```python
from build123d import *

# Parameters (mm, degrees)
BOSS_EXTRUDE1_DEPTH       = 8
SKETCH2_W                 = 5
SKETCH2_H                 = 5
LPATTERN1_COUNT           = 2
LPATTERN1_PITCH           = 20
LPATTERN1_COL_COUNT       = 2
LPATTERN1_COL_PITCH       = 20
LPATTERN2_COUNT           = 2
LPATTERN2_PITCH           = 25
LPATTERN2_COPY_1_SKETCH_W = 5
LPATTERN2_COPY_1_SKETCH_H = 5
LPATTERN2_COPY_2_SKETCH_W = 5
LPATTERN2_COPY_2_SKETCH_H = 5
SKETCH3_W                 = 30
SKETCH3_H                 = 40
CUT_EXTRUDE1_DEPTH        = 3
FILLET1_R                 = 5
CHAMFER1_SIZE             = 1
SKETCH4_R                 = 1.5
SKETCH4_R_2               = 2.5
CUT_EXTRUDE2_DEPTH        = 131.748804966
SKETCH5_W                 = 12
SKETCH5_H                 = 12
CUT_EXTRUDE3_DEPTH        = 3
FILLET2_R                 = 5


with BuildPart() as part:
    # Sketch1 → Boss-Extrude1 (new body)
    with BuildSketch(Plane(origin=(0, 0, 0), x_dir=(1, 0, 0), z_dir=(0, 1, 0))):
        Polygon((-37.5, 0), (37.5, 0), (37.5, 100), (0, 125), (-37.5, 100), align=None)
    extrude(amount=BOSS_EXTRUDE1_DEPTH)

    # Sketch2 → Revolve1 (revolve)
    with BuildSketch(Plane(origin=(0, 0, 0), x_dir=(0, 0, -1), z_dir=(1, 0, 0)), mode=Mode.PRIVATE) as revolve1_sk:
        with Locations((17.5, 10.5)):
            Rectangle(SKETCH2_W, SKETCH2_H)
    revolve1 = revolve(revolve1_sk.sketch.rotate(Axis((0, 8, -20), (0, 1, 0)), 180), axis=Axis((0, 8, -20), (0, 1, 0)))

    # LPattern1: Revolve1 ×2
    with Locations(*[(-i * LPATTERN1_PITCH, 0, 0) for i in range(1, LPATTERN1_COUNT)]):
        add(revolve1)

    # LPattern1 col: Revolve1 ×2
    with Locations(*[(i * LPATTERN1_COL_PITCH, 0, 0) for i in range(1, LPATTERN1_COL_COUNT)]):
        add(revolve1)

    # LPattern2: Revolve1 ×2
    with Locations(*[(0, 0, -i * LPATTERN2_PITCH) for i in range(1, LPATTERN2_COUNT)]):
        add(revolve1)

    # LPattern2 copy 1 sketch → LPattern2 copy 1 (revolve)
    with BuildSketch(Plane(origin=(-20, 0, -25), x_dir=(0, 0, -1), z_dir=(1, 0, 0))):
        with Locations((17.5, 10.5)):
            Rectangle(LPATTERN2_COPY_1_SKETCH_W, LPATTERN2_COPY_1_SKETCH_H)
    revolve(axis=Axis((-20, 8, -45), (0, 1, 0)))

    # LPattern2 copy 2 sketch → LPattern2 copy 2 (revolve)
    with BuildSketch(Plane(origin=(20, 0, -25), x_dir=(0, 0, -1), z_dir=(1, 0, 0))):
        with Locations((17.5, 10.5)):
            Rectangle(LPATTERN2_COPY_2_SKETCH_W, LPATTERN2_COPY_2_SKETCH_H)
    revolve(axis=Axis((20, 8, -45), (0, 1, 0)))

    # Sketch3 → Cut-Extrude1 (cut)
    with BuildSketch(Plane(origin=(0, 8, 0), x_dir=(1, 0, 0), z_dir=(0, 1, 0))):
        with Locations((0, 80)):
            Rectangle(SKETCH3_W, SKETCH3_H)
    extrude(amount=-CUT_EXTRUDE1_DEPTH, mode=Mode.SUBTRACT)

    # Fillet1
    fillet1_edges = [part.edges().sort_by_distance(p)[0] for p in [
        (-15, 6.5, -60),
        (-15, 6.5, -100),
        (15, 6.5, -100),
        (15, 6.5, -60),
    ]]
    fillet(fillet1_edges, radius=FILLET1_R)

    # Chamfer1
    chamfer1_edges = [part.edges().sort_by_distance(p)[0] for p in [
        (18.75, 8, -112.5),
        (-18.75, 8, -112.5),
        (0, 13, -15),
        (20, 13, -15),
        (-37.5, 8, -50),
        (-20, 13, -15),
        (0, 8, 0),
        (0, 13, -40),
        (20, 13, -50),
        (-20, 13, -50),
        (37.5, 8, -50),
        (15, 8, -80),
        (0, 8, -60),
        (0, 8, -100),
        (-15, 8, -80),
        (13.535533906, 8, -61.464466094),
        (13.535533906, 8, -98.535533906),
        (-13.535533906, 8, -61.464466094),
        (-13.535533906, 8, -98.535533906),
    ]]
    chamfer(chamfer1_edges, length=CHAMFER1_SIZE)

    # Sketch4 → Cut-Extrude2 (cut, through all)
    with BuildSketch(Plane(origin=(0, 5, 0), x_dir=(1, 0, 0), z_dir=(0, 1, 0))):
        with Locations(Location((0, 90, 0), (0, 0, 270))):
            Circle(SKETCH4_R)
        with Locations(Location((0, 80, 0), (0, 0, 270))):
            Circle(SKETCH4_R_2)
        with Locations(Location((0, 70, 0), (0, 0, 270))):
            Circle(SKETCH4_R)
    extrude(amount=-CUT_EXTRUDE2_DEPTH, mode=Mode.SUBTRACT)

    # Sketch5 → Cut-Extrude3 (cut)
    with BuildSketch(Plane(origin=(0, 5, 0), x_dir=(1, 0, 0), z_dir=(0, 1, 0))):
        with Locations((0, 80)):
            Rectangle(SKETCH5_W, SKETCH5_H)
    extrude(amount=-CUT_EXTRUDE3_DEPTH, mode=Mode.SUBTRACT)

    # Fillet2
    fillet2_edges = [part.edges().sort_by_distance(p)[0] for p in [
        (-6, 3.5, -74),
        (-6, 3.5, -86),
        (6, 3.5, -86),
        (6, 3.5, -74),
    ]]
    fillet(fillet2_edges, radius=FILLET2_R)


solid = part.part
```
Design review of the part built by this model. Coordinates are the model's own, in mm. A direction names the side the tool comes from. Coordinates: 2 decimals unless noted, no trailing zeros. Loops run counter-clockwise (first coordinate to the right, second up) from the corner with the lowest first, then second, coordinate; pieces in that order, holes last. Notation, with made-up numbers: M -1,41 L 4,41 A9 ccw 4,45 Z; hole C 2.5,21.5 d10. An arc over 180 degrees is marked long. One line per question, with ' | ' between items.
(1) We need section B-B (y = 10.5). Give the boundary of the cut face in (x, z).
Filled in:
outline: C -20,-45 d10; C -20,-20 d10; C 0,-45 d10; C 0,-20 d10; C 20,-45 d10; C 20,-20 d10
(2) Wall thickness on probe 1 along X at (y, z) = (8.5, -45); probe 2 along Z at (x, y) = (-17, 9.75); probe 3 along X at (y, z) = (3.8, -90): over which ranges is each line inside the solid? List them lowest first.
Filled in:
probe 1: x = -25 to -15, -5 to 5, 15 to 25 | probe 2: z = -49 to -41, -24 to -16 | probe 3: x = -37.5 to -1.5, 1.5 to 37.5
(3) We need section A-A (z = -90). Give the boundary of the cut face in (x, y), and give its area (3 significant figures).
Filled in:
outline: M -37.5,0 L -1.5,0 L -1.5,5 L -15,5 L -15,7 L -16,8 L -36.5,8 L -37.5,7 Z; M 1.5,0 L 37.5,0 L 37.5,7 L 36.5,8 L 16,8 L 15,7 L 15,5 L 1.5,5 Z | area: 493 mm^2
(4) Machinability: for faces 1 (the face through (37.5, 3, -49)), 2 (the face through (5, 3, -84)), which of the approach directions +Z, -Z, +X, -X, +Y, -Y give a long, thin tool a straight path to every point of the face, cutting with its end or side? Answer none if there is none.
Filled in:
face 1: +Z, -Z, +X, +Y, -Y | face 2: +Y
(5) We need section C-C (z = -45). Give the boundary of the cut face in (x, y).
Filled in:
outline: M -37.5,0 L 37.5,0 L 37.5,7 L 36.5,8 L 25,8 L 25,12 L 24,13 L 16,13 L 15,12 L 15,8 L 5,8 L 5,12 L 4,13 L -4,13 L -5,12 L -5,8 L -15,8 L -15,12 L -16,13 L -24,13 L -25,12 L -25,8 L -36.5,8 L -37.5,7 Z
(6) Draft analysis for pull direction Z (two halves, no side actions). For faces 3 (the face through (0.45, 2.54, -88.57)), 4 (the face through (-37.5, 3, -51)), 5 (the face through (19.012, 3.451, -112.325)), state which applies: released by +Z, released by -Z, zero draft, split by the parting line, or undercut.
Filled in:
face 3: undercut | face 4: zero draft | face 5: released by -Z
(7) For pin 1 Ø4 at (x, z) = (1.5, -67.5) entering from +Y; pin 2 Ø6 at (x, z) = (2.5, -78) entering from +Y; pin 3 Ø2 at (x, y) = (6.5, 7.5) entering from -Z, all flat-tipped, find the tip position at first contact; note any pin that passes through.
Filled in:
pin 1: stops at y = 5 | pin 2: stops at y = 2 | pin 3: stops at z = -121.24
(8) We need section D-D (x = 8.5). Give the boundary of the cut face in (y, z).
Filled in:
outline: M 0,-119.33 L 7,-119.33 L 8,-118.13 L 8,-101 L 7,-100 L 5,-100 L 5,-60 L 7,-60 L 8,-59 L 8,-1 L 7,0 L 0,0 Z
